from build123d import *

# Parameters (mm, degrees)
F1_DEPTH = 8.0645
F3_DEPTH = 6.5659


with BuildPart() as f1:
    # F0 (on Top) → F1 (new body)
    with BuildSketch(Plane.XY):
        with BuildLine():
            ThreePointArc((5.0038, -5.5245), (10.5283, 0), (5.0038, 5.5245))
            Line((5.0038, 5.5245), (-5.0038, 5.5245))
            ThreePointArc((-5.0038, 5.5245), (-10.5283, 0), (-5.0038, -5.5245))
            Line((-5.0038, -5.5245), (5.0038, -5.5245))
        make_face()
    extrude(amount=F1_DEPTH)

    # F2 (on face) → F3 (cut)
    with BuildSketch(Plane.XY.offset(8.0645)):
        with BuildLine():
            Line((7.90575, -4.700935), (7.90575, 4.700935))
            ThreePointArc((7.90575, 4.700935), (6.512075, 5.314622), (5.0038, 5.5245))
            Line((5.0038, 5.5245), (-5.0038, 5.5245))
            ThreePointArc((-5.0038, 5.5245), (-6.512075, 5.314622), (-7.90575, 4.700935))
            Line((-7.90575, 4.700935), (-7.90575, -4.700935))
            ThreePointArc((-7.90575, -4.700935), (-6.512075, -5.314622), (-5.0038, -5.5245))
            Line((-5.0038, -5.5245), (5.0038, -5.5245))
            ThreePointArc((5.0038, -5.5245), (6.512075, -5.314622), (7.90575, -4.700935))
        make_face()
    extrude(amount=-F3_DEPTH, mode=Mode.SUBTRACT)


solid = f1.part
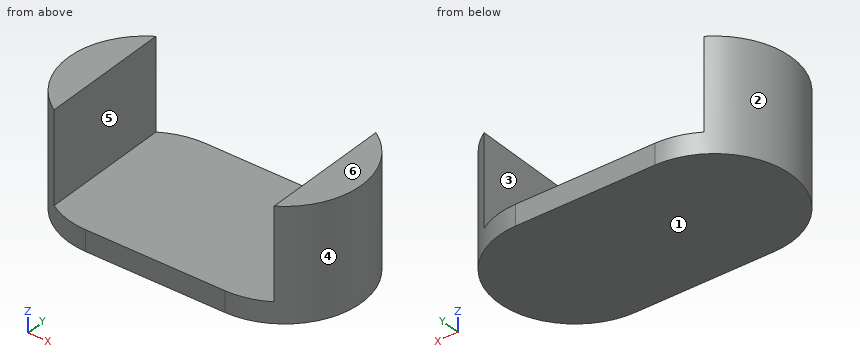
CAD build for the part. Positions are in the model's coordinates, mm. Face numbers are marked on the shaded views. A direction names the side the tool comes from. Round coordinates to 2 decimals unless told otherwise and drop trailing zeros. Loops run counter-clockwise (first coordinate to the right, second up) from the corner with the lowest first, then second, coordinate; pieces in that order, holes last.
(1) Cut at B-B (z = 4.5). Give the cut face in (x, y).
(2) Drop a flat-ended pin along its axis: pin 1 (1 mm diameter, centred on x = 6.5, y = 2.5, fed in from +Z). Give the stop position or say it passes through.
(3) Cut at D-D (z = 1.25). Give the cut face in (x, y).
(4) Cut at C-C (x = -2.5). Give the cut face in (y, z), plus the area to 3 significant figures.
(5) Which spindle directions (+Z, -Z, +X, -X, +Y, -Y) get a long thin tool onto all of the face, cutting with end or side? Do the marked faces 5 and 6. Say none if no direction does.
(6) Wall check: line 1 along X through (y, z) = (-1, 3.75); line 2 along Z through (x, y) = (-5.25, 3.75); line 3 along X through (y, z) = (3.5, 3.75). Give the ranges that are in metal, low to high.
(7) Two-plate mould, pull along X, no slides. Class the marked faces 1, 2, 3 and 4: +X half, -X half, draft (parallel to the pull), parting line (faces both ways), or undercut.
(8) Cut at A-A (y = 0). Give the cut face in (x, z), plus the area to 3 significant figures.
Findings below:
1. outline: (-7.91, -4.7) - (-7.91, 4.7) arc R5.52 ccw to start; (7.91, -4.7) arc R5.52 ccw to (7.91, 4.7) - close
2. pin 1: stops at z = 1.5
3. outline: (-5, -5.52) - (5, -5.52) arc R5.52 ccw to (5, 5.52) - (-5, 5.52) arc R5.52 ccw to start
4. outline: (-5.52, 0) - (5.52, 0) - (5.52, 1.5) - (-5.52, 1.5) - close
4. area: 16.6 mm2
5. face 5: +Z, +Y, -Y
5. face 6: +Z, +X, -X, +Y, -Y
6. line 1: x = -10.44 to -7.91, 7.91 to 10.44
6. line 2: z = 0 to 1.5
6. line 3: x = -9.28 to -7.91, 7.91 to 9.28
7. face 1: draft
7. face 2: -X half
7. face 3: undercut
7. face 4: +X half
8. outline: (-10.53, 0) - (10.53, 0) - (10.53, 8.06) - (7.91, 8.06) - (7.91, 1.5) - (-7.91, 1.5) - (-7.91, 8.06) - (-10.53, 8.06) - close
8. area: 66.0 mm2
